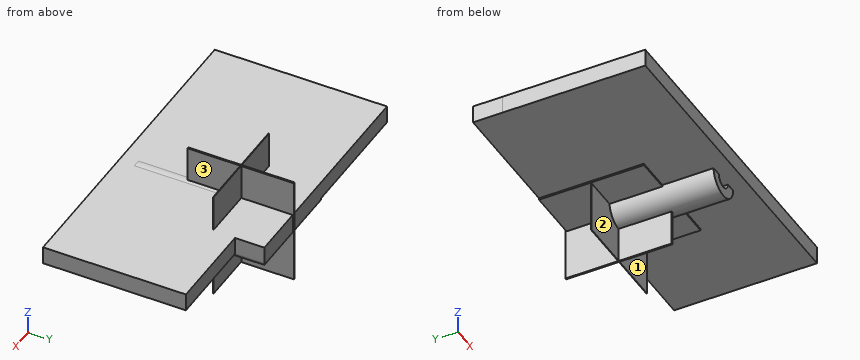
```python
from build123d import *

# Parameters (mm, degrees)
F0_R      = 25.989755
F1_DEPTH  = 148.806557
F2_R      = 12.118644
F3_DEPTH  = 78.886919
F4_R      = 12.50989
F5_DEPTH  = 42.680472
F6_W      = 151.272334
F6_H      = 149.920389
F7_DEPTH  = 2.289401
F8_W      = 151.820213
F8_H      = 153.594725
F9_DEPTH  = 2.064951
F10_W     = 148.121752
F10_H     = 153.908267
F11_DEPTH = 0.826154
F12_W     = 327.465571
F12_H     = 41.953165
F13_DEPTH = 25.4


with BuildPart() as f1:
    # F0 (on Front) → F1 (new body)
    with BuildSketch(Plane.XZ):
        Circle(F0_R)
    extrude(amount=F1_DEPTH)

    # F2 (on face) → F3 (cut)
    with BuildSketch(Plane.XZ.offset(148.806557)):
        Circle(F2_R)
    extrude(amount=-F3_DEPTH, mode=Mode.SUBTRACT)

    # F4 (on face) → F5 (join)
    with BuildSketch(Plane.XZ.offset(69.919638)):
        with Locations((-6.009842, 0)):
            Circle(F4_R)
    extrude(amount=-F5_DEPTH)

    # F6 (on Top) → F7 (join)
    with BuildSketch(Plane.XY):
        with Locations((0.205088, -0.644424)):
            Rectangle(F6_W, F6_H)
    extrude(amount=-F7_DEPTH)

    # F8 (on Right) → F9 (join)
    with BuildSketch(Plane.YZ):
        with Locations((-0.092081, -0.352483)):
            Rectangle(F8_W, F8_H)
    extrude(amount=-F9_DEPTH)

    # F10 (on Front) → F11 (join)
    with BuildSketch(Plane.XZ):
        with Locations((-0.201192, 0.494554)):
            Rectangle(F10_W, F10_H)
    extrude(amount=-F11_DEPTH)

    # F12 (on face) → F13 (join)
    with BuildSketch(Plane.XY):
        with Locations((-87.891531, 53.339188)):
            Rectangle(F12_W, F12_H)
        Polygon((206.956223, 32.362606), (75.841255, 32.362606), (-251.624316, 32.362606), (-251.624316, -171.868116), (206.956223, -171.868116), align=None)
    extrude(amount=F13_DEPTH)


solid = f1.part
```
The listing builds one solid part. Answer for the finished solid, in the listing's coordinates (mm). Face numbers are marked on the shaded views. A direction names the side the tool comes from. Give positions to 0.01 mm unless a question says otherwise; leave off trailing zeros. Loops run counter-clockwise (first coordinate to the right, second up) from the corner with the lowest first, then second, coordinate; pieces in that order, holes last. Notation, with made-up numbers: (57.5, 31) - (98.5, 31) arc R36 ccw to (98.5, 68) - close; hole circle Ø4 at (83.5, 9). An arc over 180 degrees is marked (long way). Return JSON: item names as keys, results as strings. Group by question number.
1. Find section A-A (y = -103). Write down the section's boundary in (x, z).
2. Straight lines are drawn through the part: line 1 (X direction, y = 19, z = -14.5); line 2 (Y direction, x = -16, z = 56); line 3 (Z direction, x = -174, y = -101). For each, find the intervals that lie inside material, in ascending order. Write a range as [from, to].
3. Given pin 1 Ø1.7 at (x, z) = (-1, -58) entering from -Y; pin 2 Ø4.5 at (x, y) = (-8, -73) entering from -Z; pin 3 Ø14 at (x, z) = (-93, 13) entering from +Y, each flat-ended and moving along its own axis, determine where each tip first touches the part or whether it passes through.
4. Find section C-C (x = -46.5). Write down the section's boundary in (y, z), then the cut area to 3 significant figures.
5. Which of the six approach directions +Z, -Z, +X, -X, +Y, -Y give full straight-line access (tool end or side, diameter ignored) to the marked faces 1, 2 and 3?
6. Find section D-D (y = -61). Write down the section's boundary in (x, z).
7. Find section B-B (z = 14.5). Write down the section's boundary in (x, y).
Verdict:
{
 "1": {"outline": "(-251.62, 0) - (-25.99, 0) arc R25.99 ccw to (25.99, 0) - (206.96, 0) - (206.96, 25.4) - (5.51, 25.4) arc R25.99 ccw to (-5.51, 25.4) - (-251.62, 25.4) - close; hole (-12.12, 0) arc R12.12 ccw to (12.12, 0) - close"},
 "2": {"line 1": "x = [-2.06, 0]", "line 2": "y = [0, 0.83]", "line 3": "z = [0, 25.4]"},
 "3": {"pin 1": "stops at y = -76", "pin 2": "stops at z = -25.35", "pin 3": "stops at y = 74.32"},
 "4": {"outline": "(-171.87, 0) - (-75.6, 0) - (-75.6, -2.29) - (0, -2.29) - (0, -76.46) - (0.83, -76.46) - (0.83, -2.29) - (74.32, -2.29) - (74.32, 25.4) - (0.83, 25.4) - (0.83, 77.45) - (0, 77.45) - (0, 25.4) - (-171.87, 25.4) - close", "area": "6,700 mm^2"},
 "5": {"face 1": "-Z, +X, -Y", "face 2": "-Z, -X, -Y", "face 3": "+Z, +X, -Y"},
 "6": {"outline": "(-251.62, 0) - (-75.43, 0) - (-75.43, -2.29) - (-25.89, -2.29) arc R25.99 ccw to (-2.06, -25.91) - (-2.06, -77.15) - (0, -77.15) - (0, -25.99) arc R25.99 ccw to (25.89, -2.29) - (75.84, -2.29) - (75.84, 0) - (206.96, 0) - (206.96, 25.4) - (5.51, 25.4) arc R25.99 ccw to (0, 25.99) - (0, 76.44) - (-2.06, 76.44) - (-2.06, 25.91) arc R25.99 ccw to (-5.51, 25.4) - (-251.62, 25.4) - close"},
 "7": {"outline": "(-251.62, -171.87) - (206.96, -171.87) - (206.96, 32.36) - (75.84, 32.36) - (75.84, 74.32) - (0, 74.32) - (0, 75.82) - (-2.06, 75.82) - (-2.06, 74.32) - (-251.62, 74.32) - close"}
}
